Answer from the drawing. Dimensions are ordinates in mm from the lowest x, y and z of the part. A direction names the side the tool comes from. Coordinates: 2 decimals unless noted, no trailing zeros. Write each loop counter-clockwise with the first axis right and the second up, starting at its lowest first coordinate (ties: lowest second). Pieces come first, ordered by that corner, then holes. Notation, with made-up numbers: (14.25, 17) -> (61.25, 17) arc R33 cw to (61.25, 46) -> close; hole circle Ø9 at (59.5, 13.5). An arc over 180 degrees is marked (long way). One line per item, written item: value. Start each with the question number.
1. Find section B-B, the plane y = 0.55. Write down the section's boundary in (x, z).
2. Find section A-A, the plane z = 19.5. Write down the section's boundary in (x, y).
3. Find section C-C, the plane x = 13.75. Write down the section's boundary in (y, z), and give its area (3 significant figures).
4. For the marked faces 1, 2 and 3, determine the directions among +Z, -Z, +X, -X, +Y, -Y from which every point of the face is accessible in a straight line to the end or side of a thin tool.
5. Given P1, Ø6, axis at x = 10.5, z = 17, coming from the +Y side; P2, Ø4, axis at x = 2, z = 12.5, coming from the +Y side; P3, Ø2, axis at x = 15.5, y = 1.5, coming from the +Z side, each flat-ended and moving along its own axis, determine where each tip first touches the part or whether it passes through.
6. Find section D-D, the plane y = 4.4. Write down the section's boundary in (x, z).
7. Consider line 1 along Z through (x, y) = (4.8, 0.35); line 2 along X through (y, z) = (0.75, 5.5); line 3 along Y through (x, z) = (12.5, 21.5). Determine where each line is inside the solid, lowest interval first.
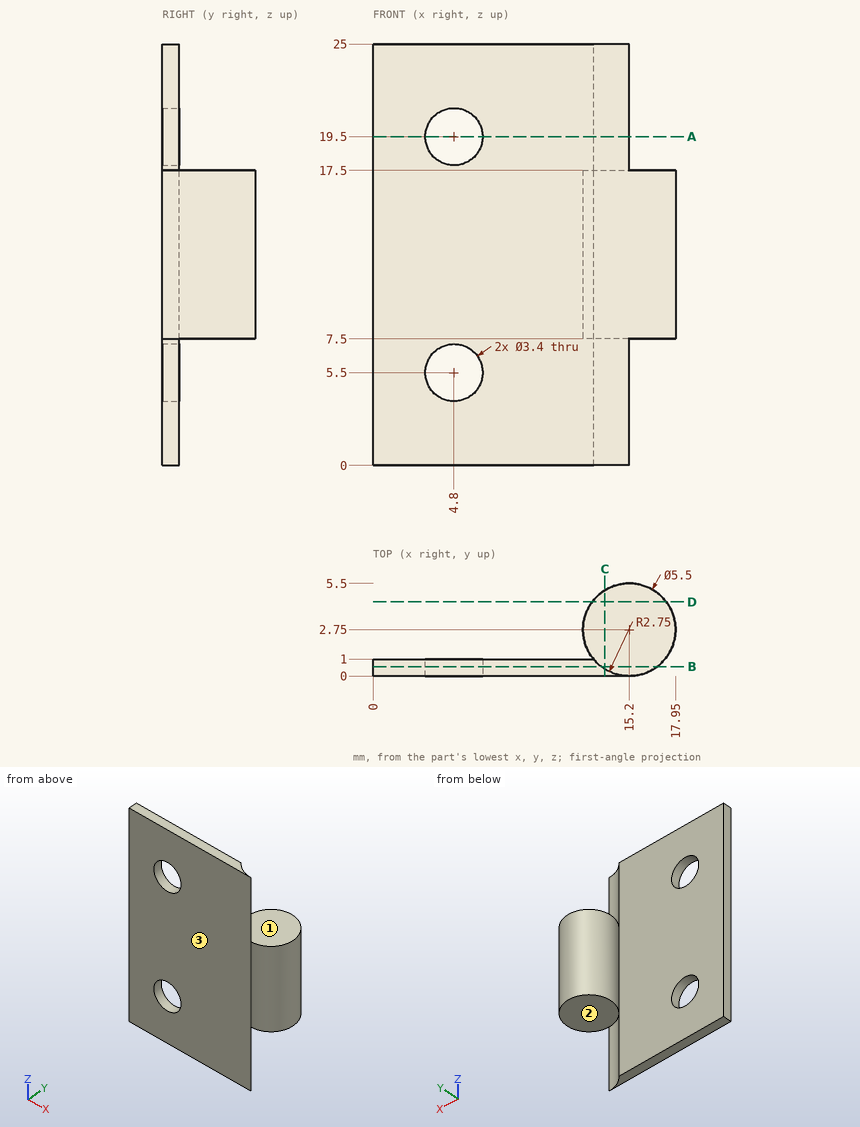
Answer block:
1. outline: (0, 0) -> (13.55, 0) -> (13.55, 7.5) -> (16.85, 7.5) -> (16.85, 17.5) -> (13.55, 17.5) -> (13.55, 25) -> (0, 25) -> close; hole circle Ø3.4 at (4.8, 5.5); hole circle Ø3.4 at (4.8, 19.5)
2. outline: (0, 0) -> (3.1, 0) -> (3.1, 1) -> (0, 1) -> close; (6.5, 0) -> (15.2, 0) arc R2.75 cw to (13.08, 1) -> (6.5, 1) -> close
3. outline: (0, 0) -> (0.41, 0) -> (0.41, 7.5) -> (5.09, 7.5) -> (5.09, 17.5) -> (0.41, 17.5) -> (0.41, 25) -> (0, 25) -> close
3. area: 57.1 mm2
4. face 1: +Z, +X, +Y
4. face 2: -Z, +X, +Y
4. face 3: +Z, -Z, +X, -X, -Y
5. P1: stops at y = 4.91
5. P2: stops at y = 1
5. P3: stops at z = 17.5
6. outline: (13, 7.5) -> (17.4, 7.5) -> (17.4, 17.5) -> (13, 17.5) -> close
7. line 1: z = 0 to 3.8, 7.2 to 17.8, 21.2 to 25
7. line 2: x = 0 to 3.1, 6.5 to 13.31
7. line 3: y = 0 to 1
